```python
from build123d import *

# Parameters (mm, degrees)
SCHIZZO1_R                   = 1
ESTRUSIONE_ESTRUSIONE1_DEPTH = 6
RACCORDO1_R                  = 8
RACCORDO2_R                  = 40
RACCORDO3_R                  = 0.5


with BuildPart() as part:
    # Schizzo1 → Estrusione-Estrusione1 (new body)
    with BuildSketch(Plane(origin=(0, 0, 0), x_dir=(0, 0, -1), z_dir=(1, 0, 0))):
        with BuildLine():
            Line((22.6, 14.5), (2.6, 14.5))
            ThreePointArc((2.6, 14.5), (-5.9, 6), (2.6, -2.5))
            Line((2.6, -2.5), (55, -2.5))
            ThreePointArc((55, -2.5), (59.829629131, 3.794095226), (52.5, 6.830127019))
            Line((52.5, 6.830127019), (48.378061008, 4))
            Line((48.378061008, 4), (22.6, 14.5))
        make_face()
        Polygon((0, 0), (0, 12), (22.6, 12), (22.6, 0), (9, 0), (9, -1), (4, -1), (4, 0), align=None, mode=Mode.SUBTRACT)
        with Locations((-2, 6)):
            Circle(SCHIZZO1_R, mode=Mode.SUBTRACT)
        with Locations((24.6, 6)):
            Circle(SCHIZZO1_R, mode=Mode.SUBTRACT)
        with Locations((55, 2.5)):
            Circle(SCHIZZO1_R, mode=Mode.SUBTRACT)
    extrude(amount=ESTRUSIONE_ESTRUSIONE1_DEPTH)

    # Raccordo1
    raccordo1_edges = [part.edges().sort_by_distance(p)[0] for p in [
        (3, 4, -48.378061008),
    ]]
    fillet(raccordo1_edges, radius=RACCORDO1_R)

    # Raccordo2
    raccordo2_edges = [part.edges().sort_by_distance(p)[0] for p in [
        (3, 14.5, -22.6),
    ]]
    fillet(raccordo2_edges, radius=RACCORDO2_R)

    # Raccordo3
    raccordo3_edges = [part.edges().sort_by_distance(p)[0] for p in [
        (3, 0, -22.6),
        (3, 0, 0),
        (3, 12, 0),
        (3, 12, -22.6),
        (3, 0, -4),
        (3, -1, -4),
        (3, -1, -9),
        (3, 0, -9),
    ]]
    fillet(raccordo3_edges, radius=RACCORDO3_R - 0.0001)  # a hair under: the kernel refuses the full size


solid = part.part
```
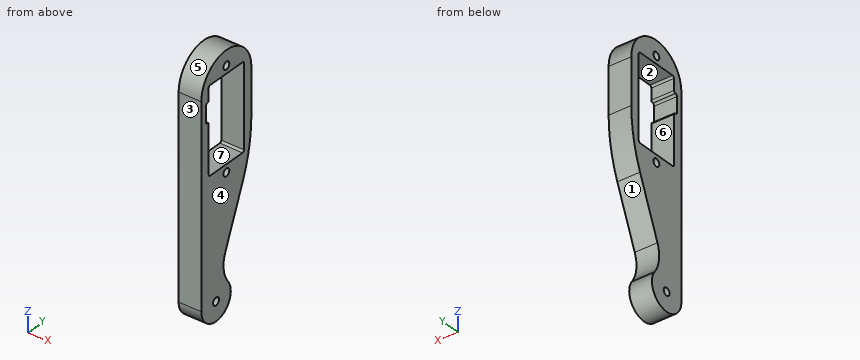
Verification items for the finished model (mm, model axes). Face numbers are marked on the shaded views. A direction names the side the tool comes from. Coordinates: 2 decimals unless noted, no trailing zeros. Loops run counter-clockwise (first coordinate to the right, second up) from the corner with the lowest first, then second, coordinate; pieces in that order, holes last. Notation, with made-up numbers: (42.5, 13.25) - (54.5, 13.25) arc R24 cw to (54.5, 28.25) - close; hole circle Ø5 at (66, 3). An arc over 180 degrees is marked (long way). Return JSON: item names as keys, results as strings.
1. Go/stop test with flat-tipped pins: pin 1 (6 mm diameter, centred on y = 12, z = -20.5, fed in from -X); pin 2 (2 mm diameter, centred on x = 5, y = 4, fed in from +Z); pin 3 (4 mm diameter, centred on y = 11.5, z = -37.5, fed in from +X); pin 4 (3 mm diameter, centred on x = 4, z = -0.5, fed in from +Y). Record where each tip stops, or that it passes through.
Established:
{"pin 1": "stops at x = 0", "pin 2": "stops at z = 5.84", "pin 3": "passes through", "pin 4": "stops at y = 14.48"}
2. Mould release check, pull along Y, two halves, no side actions. Record for the marked faces 4, 5, 6 and 7: +Y half, -Y half, draft (parallel to the pull), parting line (faces both ways), or undercut.
Established:
{"face 4": "draft", "face 5": "parting line", "face 6": "undercut", "face 7": "undercut"}
3. Section check B-B, the plane z = -24.6. Record the boundary of the cut face in (x, y), then the cut area to 3 significant figures.
Established:
{"outline": "(0, -2.5) - (6, -2.5) - (6, 5) - (0, 5) - close; (0, 7) - (6, 7) - (6, 13.27) - (0, 13.27) - close", "area": "82.6 mm2"}
4. Section check D-D, the plane y = 10.5. Record the boundary of the cut face in (x, z), then the cut area to 3 significant figures.
Established:
{"outline": "(0, -32.42) - (6, -32.42) - (6, -22.6) - (0, -22.6) - close; (0, 0) - (6, 0) - (6, 4.61) - (0, 4.61) - close", "area": "86.6 mm2"}
5. Section check C-C, the plane y = 2.5. Record the boundary of the cut face in (x, z).
Established:
{"outline": "(0, -60) - (6, -60) - (6, -56) - (0, -56) - close; (0, -54) - (6, -54) - (6, -22.6) - (0, -22.6) - close; (0, 0) - (6, 0) - (6, 5.15) - (0, 5.15) - close"}
6. Tool access check on the marked faces 1, 2 and 3. Record the directions out of +Z, -Z, +X, -X, +Y, -Y that give a thin tool (end or side, any length) a straight path to the whole face; none if there is none.
Established:
{"face 1": "+X, -X, +Y", "face 2": "+X, -X", "face 3": "+Z, -Z, +X, -X, -Y"}
7. Thickness scan on L1, parallel to Y at x = 1.4, z = -15.5; L2, parallel to Y at x = 5.25, z = -5.5; L3, parallel to Y at x = 4.05, z = -30. Record the ranges inside material, lowest first.
Established:
{"L1": "y = -2.5 to 0, 12 to 14.49", "L2": "y = -2.5 to -1, 12 to 14.5", "L3": "y = -2.5 to 11.49"}
8. Section check A-A, the plane x = 0.7. Count the separate pieces of the cut face and the enclosed holes in it, then the cut area to 3 significant figures.
Established:
{"separate pieces": "1", "enclosed holes": "4", "area": "566 mm2"}
